Here's how the part is built. I have some questions about the finished solid (model axes, mm). A direction names the side the tool comes from. Give positions to 0.01 mm unless a question says otherwise; leave off trailing zeros. Write each loop counter-clockwise with the first axis right and the second up, starting at its lowest first coordinate (ties: lowest second). Pieces come first, ordered by that corner, then holes. Notation, with made-up numbers: (58, 26) - (80, 26) arc R20 cw to (80, 60) - close; hole circle Ø3 at (12, 22.25). An arc over 180 degrees is marked (long way). Use one line per item in the form item = value. Start each with the question number.
from build123d import *

# Parameters (mm, degrees)
SKETCH1_W           = 19.338503776
SKETCH1_H           = 3.175
BOSS_EXTRUDE1_DEPTH = 3.175


with BuildPart() as part:
    # Sketch1 → Boss-Extrude1 (new body)
    with BuildSketch(Plane.XY):
        Polygon((-96.911258203, 47.780766243), (-46.911258203, 47.780766243), (-46.911258203, 39.580766243), (-50.086258203, 39.580766243), (-50.086258203, 34.580766243), (-52.911258203, 34.580766243), (-52.911258203, 36.780766243), (-55.911258203, 36.780766243), (-55.911258203, 34.580766243), (-57.411258203, 34.580766243), (-57.411258203, 30.980766243), (-55.911258203, 30.980766243), (-55.911258203, 28.780766243), (-52.911258203, 28.780766243), (-52.911258203, 30.980766243), (-50.086258203, 30.980766243), (-50.086258203, 25.980766243), (-46.911258203, 25.980766243), (-46.911258203, 17.780766243), (-96.911258203, 17.780766243), align=None)
        with Locations((-70.694345596, 21.182701237)):
            Rectangle(SKETCH1_W, SKETCH1_H, mode=Mode.SUBTRACT)
    extrude(amount=BOSS_EXTRUDE1_DEPTH)


solid = part.part
1. We'd pull the mould along X, two halves only. Please class faces 4 (the face through (-57, 34.581, 2)), 5 (the face through (-50.086, 37, 2)), 6 (the face through (-54, 28.781, 2)): pulls with the +X half, pulls with the -X half, needs draft (parallel to the pull), parting line crosses it, or undercut.
2. Please list where these lines run through material, in increasing order: line 1 (Y direction, x = -78.5, z = 2.35); line 2 (Y direction, x = -56, z = 0.95); line 3 (X direction, y = 20, z = 2.2).
3. For P1, Ø1.6, axis at y = 33, z = 1, coming from the +X side; P2, Ø1.8, axis at y = 35.5, z = 1.5, coming from the +X side, each with a flat end and sliding along its axis, tell me the tip position at first contact or that it passes through.
4. I want a section at C-C, the plane x = -51.5. List the corners of the cut face in (y, z) for me (3 decimals), then the cut area to 3 significant figures.
5. For faces 1 (the face through (-61.025, 21, 2)), 2 (the face through (-46.911, 22, 2)), 3 (the face through (-57, 30.981, 2)), which set-ups out of +Z, -Z, +X, -X, +Y, -Y let a thin tool reach every point of the face, with its end or its side?
6. I want a section at D-D, the plane y = 34. List the corners of the cut face in (x, z) for me (3 decimals), then the cut area to 3 significant figures.
7. I want a section at B-B, the plane z = 2.1. List the corners of the cut face in (x, y) for me, then the cut area to 3 significant figures.
8. I want a section at A-A, the plane x = -73.5. List the corners of the cut face in (y, z) for me (3 decimals), then the cut area to 3 significant figures.
Result sheet:
q1.face_4 = needs draft
q1.face_5 = pulls with the +X half
q1.face_6 = undercut
q2.line_1 = 17.78 to 19.6, 22.77 to 47.78
q2.line_2 = 17.78 to 30.98, 34.58 to 47.78
q2.line_3 = -96.91 to -80.36, -61.03 to -46.91
q3.P1 = -57.41
q3.P2 = -50.09
q4.outline = (17.781, 0) - (30.981, 0) - (30.981, 3.175) - (17.781, 3.175) - close; (34.581, 0) - (47.781, 0) - (47.781, 3.175) - (34.581, 3.175) - close
q4.area = 83.8 mm2
q5.face_1 = +Z, -Z
q5.face_2 = +Z, -Z, +X, +Y, -Y
q5.face_3 = +Z, -Z, +X
q6.outline = (-96.911, 0) - (-57.411, 0) - (-57.411, 3.175) - (-96.911, 3.175) - close
q6.area = 125 mm2
q7.outline = (-96.91, 17.78) - (-46.91, 17.78) - (-46.91, 25.98) - (-50.09, 25.98) - (-50.09, 30.98) - (-52.91, 30.98) - (-52.91, 28.78) - (-55.91, 28.78) - (-55.91, 30.98) - (-57.41, 30.98) - (-57.41, 34.58) - (-55.91, 34.58) - (-55.91, 36.78) - (-52.91, 36.78) - (-52.91, 34.58) - (-50.09, 34.58) - (-50.09, 39.58) - (-46.91, 39.58) - (-46.91, 47.78) - (-96.91, 47.78) - close; hole (-80.36, 19.6) - (-61.03, 19.6) - (-61.03, 22.77) - (-80.36, 22.77) - close
q7.area = 1,360 mm2
q8.outline = (17.781, 0) - (19.595, 0) - (19.595, 3.175) - (17.781, 3.175) - close; (22.77, 0) - (47.781, 0) - (47.781, 3.175) - (22.77, 3.175) - close
q8.area = 85.2 mm2
